The listing builds one solid part. Answer for the finished solid, in the listing's coordinates (mm). Round coordinates to 2 decimals unless told otherwise and drop trailing zeros. Loops run counter-clockwise (first coordinate to the right, second up) from the corner with the lowest first, then second, coordinate; pieces in that order, holes last. Notation, with made-up numbers: (36, -33) - (40, -33) arc R20 ccw to (40, -1) - close; hole circle Ø5 at (15.25, -15). An arc over 180 degrees is marked (long way). One line per question, with ' | ' between items. Start each with the question number.
Autodesk Inventor part; units mm, degrees
ref_plane "YZ Plane" through (0, 0, 0) normal (1, 0, 0) x (0, 1, 0)
ref_plane "XZ Plane" through (0, 0, 0) normal (0, 1, 0) x (-1, 0, 0)
ref_plane "XY Plane" through (0, 0, 0) normal (0, 0, 1) x (1, 0, 0)
sketch "Sketch1" plane through (0, 0, 0) normal (0, 1, 0) x (-1, 0, 0)
  line L0 (0, 0) -> (508, 0)
  line L1 (508, 0) -> (508, 584.2)
  line L2 (508, 584.2) -> (0, 584.2)
  line L3 (0, 584.2) -> (0, 0)
  dimension "d0" = 508
  dimension "d1" = 584.2
extrude "Extrusion1" add sketch "Sketch1" along normal blind 6.35
sketch "Sketch2" plane through (0, 0, 0) normal (0, -1, 0) x (1, 0, 0)
  line L0 (-508, 584.2) -> (-355.6, 584.2)
  line L1 (-355.6, 584.2) -> (-355.6, 520.7)
  line L2 (-355.6, 520.7) -> (-508, 520.7)
  line L3 (-508, 520.7) -> (-508, 584.2)
  line L4 (0, 584.2) -> (-152.4, 584.2)
  line L5 (-152.4, 584.2) -> (-152.4, 520.7)
  line L6 (-152.4, 520.7) -> (0, 520.7)
  line L7 (0, 520.7) -> (0, 584.2)
  line L8 (-508, 0) -> (-355.6, 0)
  line L9 (-355.6, 0) -> (-355.6, 63.5)
  line L10 (-355.6, 63.5) -> (-508, 63.5)
  line L11 (-508, 63.5) -> (-508, 0)
  line L12 (0, 0) -> (-152.4, 0)
  line L13 (-152.4, 0) -> (-152.4, 63.5)
  line L14 (-152.4, 63.5) -> (0, 63.5)
  line L15 (0, 63.5) -> (0, 0)
  dimension "d4" = 152.4
  dimension "d5" = 63.5
  dimension "d6" = 152.4
  dimension "d7" = 63.5
  dimension "d8" = 152.4
  dimension "d9" = 63.5
  dimension "d10" = 152.4
  dimension "d11" = 63.5
extrude "Extrusion2" cut sketch "Sketch2" against normal through all
sketch "Sketch5" plane through (0, 0, 0) normal (0, -1, 0) x (1, 0, 0)
  line L0 (-152.4, 63.5) -> (0, 63.5)
  line L1 (0, 520.7) -> (0, 63.5)
  line L2 (-508, 520.7) -> (-419.1, 520.7)
  line L3 (-419.1, 520.7) -> (-419.1, 431.8)
  line L4 (-419.1, 431.8) -> (-508, 431.8)
  line L5 (-508, 431.8) -> (-508, 520.7)
  line L6 (0, 520.7) -> (-88.9, 520.7)
  line L7 (-88.9, 520.7) -> (-88.9, 431.8)
  line L8 (-88.9, 431.8) -> (0, 431.8)
  line L9 (0, 431.8) -> (0, 520.7)
  line L10 (-508, 63.5) -> (-419.1, 63.5)
  line L11 (-419.1, 63.5) -> (-419.1, 152.4)
  line L12 (-419.1, 152.4) -> (-508, 152.4)
  line L13 (-508, 152.4) -> (-508, 63.5)
  line L14 (0, 63.5) -> (-88.9, 63.5)
  line L15 (-88.9, 63.5) -> (-88.9, 152.4)
  line L16 (-88.9, 152.4) -> (0, 152.4)
  line L17 (0, 152.4) -> (0, 63.5)
  point P0 (0, 0)
  dimension "d24" = 88.9
  dimension "d25" = 88.9
  dimension "d26" = 88.9
  dimension "d27" = 88.9
  dimension "d28" = 88.9
  dimension "d29" = 88.9
  dimension "d30" = 88.9
  dimension "d31" = 88.9
extrude "Extrusion4" cut sketch "Sketch5" against normal blind 6.35
properties part number "Belly Board" material "ABS Plastic"
(1) Find section C-C on x = -126. Write down the section's boundary in (y, z).
(2) Find section A-A on y = 4. Write down the section's boundary in (x, z), plus the area to 3 significant figures.
(3) Find section B-B on z = 91.5. Write down the section's boundary in (x, y), plus the area to 3 significant figures.
(4) Each of these flat-tipped pins is pushed along its axis until it touches: P1, Ø1.9, axis at y = 3, z = 538.5, coming from the +X side; P2, Ø1.9, axis at x = -481, y = 3.5, coming from the -Z side; P3, Ø3, axis at y = 4.5, z = 478.5, coming from the +X side. Where does it stop, or does it pass through?
(5) Consider L1, parallel to Z at x = -393, y = 1.75; L2, parallel to Z at x = -65, y = 1; L3, parallel to X at y = 4.75, z = 82. Determine where each line is inside the solid, lowest interval first.
Answer below:
1) outline: (0, 63.5) - (6.35, 63.5) - (6.35, 520.7) - (0, 520.7) - close
2) outline: (-508, 152.4) - (-419.1, 152.4) - (-419.1, 63.5) - (-355.6, 63.5) - (-355.6, 0) - (-152.4, 0) - (-152.4, 63.5) - (-88.9, 63.5) - (-88.9, 152.4) - (0, 152.4) - (0, 431.8) - (-88.9, 431.8) - (-88.9, 520.7) - (-152.4, 520.7) - (-152.4, 584.2) - (-355.6, 584.2) - (-355.6, 520.7) - (-419.1, 520.7) - (-419.1, 431.8) - (-508, 431.8) - close | area: 226,000 mm2
3) outline: (-419.1, 0) - (-88.9, 0) - (-88.9, 6.35) - (-419.1, 6.35) - close | area: 2,100 mm2
4) P1: x = -152.4 | P2: z = 152.4 | P3: x = -88.9
5) L1: 63.5 to 520.7 | L2: 152.4 to 431.8 | L3: -419.1 to -88.9
